```python
from build123d import *

# Parameters (mm, degrees)
SWEEP1_PROFILE_R   = 12.5
SKETCH8_R          = 12.5
CUT_EXTRUDE3_DEPTH = 21
SKETCH2_R          = 12.5
CUT_EXTRUDE5_DEPTH = 13


with BuildPart() as part:
    # Sweep1: sweep along a path in Sketch1
    with BuildLine(Plane.XY) as sweep1_path:
        Line((0, 0), (0, 830))
        ThreePointArc((0, 830), (-14.644660941, 865.355339059), (-50, 880))
        Line((-50, 880), (-190, 880))
    # Sweep1 profile (on start of the path) → Sweep1 (sweep)
    with BuildSketch(Plane.ZX):
        Circle(SWEEP1_PROFILE_R)
    sweep(path=sweep1_path.line)

    # Sketch8 → Cut-Extrude3 (cut)
    with BuildSketch(Plane(origin=(0, 0, 0), x_dir=(0, 0, -1), z_dir=(1, 0, 0))):
        with Locations((0, 655.01)):
            Circle(SKETCH8_R)
        with Locations((0, 375.5)):
            Circle(SKETCH8_R)
    extrude(amount=CUT_EXTRUDE3_DEPTH, mode=Mode.SUBTRACT)

    # Sketch2 → Cut-Extrude5 (cut)
    with BuildSketch(Plane.XY):
        with Locations((0, 182.5)):
            Circle(SKETCH2_R)
    extrude(amount=-CUT_EXTRUDE5_DEPTH, mode=Mode.SUBTRACT)


solid = part.part
```
For this review, take the finished solid that the model builds, in its own axes (mm). A direction names the side the tool comes from. Round coordinates to 2 decimals unless told otherwise and drop trailing zeros. Order: outer loops, then holes, each group sorted by start corner. A loop starts at its lowest first (then second) coordinate and runs counter-clockwise, first axis right, second up. Notation, with made-up numbers: (50.5, 23.5) -> (83.5, 23.5) arc R20 ccw to (83.5, 37.5) -> close; hole circle Ø4 at (8.25, 70.5). An arc over 180 degrees is marked (long way). Use a Markdown table: item, result.
Item 1: Take a section at C-C (x = -117). State the section outline as (y, z) points.
Resolved:
| item | result |
|---|---|
| outline | circle Ø25 at (880, 0) |
Item 2: For line 1 along Y through (x, z) = (-156.5, 0.5); line 2 along X through (y, z) = (554, 1); line 3 along X through (y, z) = (454.5, -1.5), list the stretches that pass through material, from the lowest coordinate up. Write a range as [from, to].
Resolved:
| item | result |
|---|---|
| line 1 | y = [867.51, 892.49] |
| line 2 | x = [-12.46, 12.46] |
| line 3 | x = [-12.41, 12.41] |
Item 3: For pin 1 (1 mm diameter, centred on y = 100, z = 0, fed in from -X); pin 2 (12 mm diameter, centred on y = 107, z = -7.5, fed in from +X); pin 3 (12.5 mm diameter, centred on y = 651, z = 1, fed in from +X), all flat-tipped, find the tip position at first contact; note any pin that passes through.
Resolved:
| item | result |
|---|---|
| pin 1 | stops at x = -12.5 |
| pin 2 | stops at x = 12.41 |
| pin 3 | stops at x = 0 |
Item 4: Machinability: for faces 4 (the flat face through (0, 183, 0)), 5 (the cylindrical face through (3.755, 420.81, 11.923)), 6 (the flat face through (0, 376, 0)), which of the approach directions +Z, -Z, +X, -X, +Y, -Y give a long, thin tool a straight path to every point of the face, cutting with its end or side? Answer none if there is none.
Resolved:
| item | result |
|---|---|
| face 4 | -Z |
| face 5 | -Y |
| face 6 | +X |
Item 5: Take a section at A-A (z = 7.5). State the section outline as (x, y) points.
Resolved:
| item | result |
|---|---|
| outline | (-190, 870) -> (-50, 870) arc R40 cw to (-10, 830) -> (-10, 0) -> (10, 0) -> (10, 365.5) -> (0, 365.5) -> (0, 385.5) -> (10, 385.5) -> (10, 645.01) -> (0, 645.01) -> (0, 665.01) -> (10, 665.01) -> (10, 830) arc R60 ccw to (-50, 890) -> (-190, 890) -> close |
Item 6: Take a section at B-B (y = 734). State the section outline as (x, z) points.
Resolved:
| item | result |
|---|---|
| outline | circle Ø25 at (0, 0) |
Item 7: Draft analysis for pull direction Y (two halves, no side actions). For faces 1 (the flat face through (0, 0, 0)), 2 (the flat face through (0, 655, 0)), 3 (the cylindrical face through (-120.98, 867.797, -2.71)), state which applies: +Y half, -Y half, draft (parallel to the pull), parting line (faces both ways), or undercut.
Resolved:
| item | result |
|---|---|
| face 1 | -Y half |
| face 2 | undercut |
| face 3 | parting line |
